The listing builds one solid part. Answer for the finished solid, in the listing's coordinates (mm). A direction names the side the tool comes from. Give positions to 0.01 mm unless a question says otherwise; leave off trailing zeros. Order: outer loops, then holes, each group sorted by start corner. A loop starts at its lowest first (then second) coordinate and runs counter-clockwise, first axis right, second up. Notation, with made-up numbers: (-30, 81) - (25, 81) arc R23 ccw to (25, 99) - close; hole circle Ø4 at (88, 18). An arc over 180 degrees is marked (long way). Write each question's results on one line, items separated by ' | '. Start each with the question number.
1. Flat-ended cylindrical pins translate along their axes: pin 1 (12 mm diameter, centred on x = -8.5, y = -22, fed in from +Z); pin 2 (8 mm diameter, centred on x = -15, z = -6, fed in from +Y); pin 3 (3 mm diameter, centred on y = 13.5, z = 1, fed in from +X); pin 4 (4 mm diameter, centred on y = 1, z = -5.5, fed in from -X). Find the tip coordinate at first contact, or state that the pin passes through.
2. Section B-B (y = 0) is taken. Give the vertices of the cut face in (x, z).
3. Section A-A (x = 0) is taken. Give the vertices of the cut face in (y, z).
4. Section C-C (z = 4) is taken. Give the vertices of the cut face in (x, y).
5. Determine the mould class of faces 1 (the face through (32.907, 10.363, 3.458)), 2 (the face through (25.03, -22.51, 7)), 3 (the face through (30.5, -12.6, -0.9)) for opening direction X: released by +X, released by -X, zero draft, split by the parting line, or undercut.
6. Which of the six approach directions +Z, -Z, +X, -X, +Y, -Y give full straight-line access (tool end or side, diameter ignored) to faces 4 (the face through (19, 30, 0)), 5 (the face through (-1, -1, -10)), 6 (the face through (-0.434, 34.941, -6.452))?
7. Find the intervals of material crossed by L1, parallel to Y at x = 0, z = -1.5; L2, parallel to Z at x = 0, y = 34.95; L3, parallel to Z at x = 29.5, y = -13, in increasing order.
8. Section D-D (z = -4.5) is taken. Give the vertices of the cut face in (x, y).
from build123d import *

# Parameters (mm, degrees)
SKETCH_R        = 34.5
PAD_DEPTH       = 7
SKETCH001_R     = 37
PAD001_DEPTH    = 10
SKETCH002_R     = 33
POCKET_DEPTH    = 16
SKETCH003_R     = 2
POCKET001_DEPTH = 80
FILLET_R        = 0.5
CHAMFER_SIZE    = 0.5


with BuildPart() as part:
    # Sketch → Pad (new body)
    with BuildSketch(Plane.XY):
        Circle(SKETCH_R)
    extrude(amount=PAD_DEPTH)

    # Sketch001 (on Face2 of Pad) → Pad001 (join)
    with BuildSketch(Plane(origin=(0, 0, 0), x_dir=(1, 0, 0), z_dir=(0, 0, -1))):
        Circle(SKETCH001_R)
    extrude(amount=PAD001_DEPTH)

    # Sketch002 (on Face5 of Pad001) → Pocket (cut)
    with BuildSketch(Plane.XY.offset(7)):
        Circle(SKETCH002_R)
    extrude(amount=-POCKET_DEPTH, mode=Mode.SUBTRACT)

    # Sketch003 → Pocket001 (cut)
    with BuildSketch(Plane.XZ):
        with Locations((0, -4.5)):
            Circle(SKETCH003_R)
    extrude(amount=-POCKET001_DEPTH, mode=Mode.SUBTRACT)

    # Fillet
    fillet_edges = [part.edges().sort_by_distance(p)[0] for p in [
        (-33, 0, 7),
        (-34.5, 0, 0),
        (-37, 0, 0),
        (-37, 0, -10),
        (-33, 0, -9),
    ]]
    fillet(fillet_edges, radius=FILLET_R)

    # Chamfer
    chamfer_edges = [part.edges().sort_by_distance(p)[0] for p in [
        (-34.5, 0, 7),
    ]]
    chamfer(chamfer_edges, length=CHAMFER_SIZE)


solid = part.part
Reported:
1) pin 1: z = -9 | pin 2: y = 35.33 | pin 3: x = 34.69 | pin 4: x = -37
2) outline: (-37, -9.5) arc R0.5 ccw to (-36.5, -10) - (36.5, -10) arc R0.5 ccw to (37, -9.5) - (37, -0.5) arc R0.5 ccw to (36.5, 0) - (35, 0) arc R0.5 cw to (34.5, 0.5) - (34.5, 6.5) - (34, 7) - (33.5, 7) arc R0.5 ccw to (33, 6.5) - (33, -8.5) arc R0.5 cw to (32.5, -9) - (-32.5, -9) arc R0.5 cw to (-33, -8.5) - (-33, 6.5) arc R0.5 ccw to (-33.5, 7) - (-34, 7) - (-34.5, 6.5) - (-34.5, 0.5) arc R0.5 cw to (-35, 0) - (-36.5, 0) arc R0.5 ccw to (-37, -0.5) - close
3) outline: (-37, -9.5) arc R0.5 ccw to (-36.5, -10) - (36.5, -10) arc R0.5 ccw to (37, -9.5) - (37, -6.5) - (33, -6.5) - (33, -8.5) arc R0.5 cw to (32.5, -9) - (-32.5, -9) arc R0.5 cw to (-33, -8.5) - (-33, 6.5) arc R0.5 ccw to (-33.5, 7) - (-34, 7) - (-34.5, 6.5) - (-34.5, 0.5) arc R0.5 cw to (-35, 0) - (-36.5, 0) arc R0.5 ccw to (-37, -0.5) - close; (33, -2.5) - (37, -2.5) - (37, -0.5) arc R0.5 ccw to (36.5, 0) - (35, 0) arc R0.5 cw to (34.5, 0.5) - (34.5, 6.5) - (34, 7) - (33.5, 7) arc R0.5 ccw to (33, 6.5) - close
4) outline: circle Ø69 at (0, 0); hole circle Ø66 at (0, 0)
5) face 1: split by the parting line | face 2: zero draft | face 3: undercut
6) face 4: +Z | face 5: -Z, +X, -X, +Y, -Y | face 6: +Y
7) L1: -37 to -33, 33 to 37 | L2: -10 to -6.5, -2.5 to 0 | L3: -10 to -9
8) outline: (-2, 32.94) - (-2, 36.95) arc R37 ccw (long way) to (2, 36.95) - (2, 32.94) arc R33 cw (long way) to start
